Source: CAD feature listing. Evaluate the final solid. Frame: model axes, mm. A direction names the side the tool comes from. Round coordinates to 2 decimals unless told otherwise and drop trailing zeros. Loops run counter-clockwise (first coordinate to the right, second up) from the corner with the lowest first, then second, coordinate; pieces in that order, holes last.
(1) Material intervals for probe 1 along Z at (x, y) = (0, -2.9); probe 2 along X at (y, z) = (-1.55, -13.5); probe 3 along X at (y, z) = (-4.95, -16), sorted ascending.
(2) Section C-C, the plane x = -1.5. Return the cut outline in (y, z), plus the area to 3 significant figures.
(3) First-contact query: pin 1 Ø10 at (x, z) = (-16, -13.5) entering from -Y; pin 2 Ø10 at (x, z) = (-31, -17.5) entering from -Y; pin 3 Ø1 at (x, y) = (3, -2.5) entering from +Z; pin 4 Ø20 at (x, z) = (0, 0) entering from -Y. Flat tips, straight axial feed; report the tip coordinate or a pass-through.
(4) Section B-B, the plane y = -3. Return the cut outline in (x, z).
(5) Mould query, pull axis Z, two halves, no side actions, for faces 4 (the flat face through (11.4, -3, -23.9)), 5 (the flat face through (9, -6, -9)), 6 (the cylindrical face through (-2.38, -2.96, -10.74)). Classes: pulls with the +Z half, pulls with the -Z half, needs draft (parallel to the pull), parting line crosses it, or undercut.
(6) Section D-D, the plane x = 33.5. Return the cut outline in (y, z) (3 decimals), plus the area to 3 significant figures.
(7) Section A-A, the plane z = 0. Return the cut outline in (x, y).
(8) Set-up query: faces 1 (the flat face through (18, -1, -10)), 2 (the flat face through (-15, -3, 22)), 3 (the flat face through (15, -3, 22)). Return all of +Z, -Z, +X, -X, +Y, -Y with unobstructed straight access to the full face (end or side cutting, diameter ignored); none if empty.
```python
from build123d import *

# Parameters (mm, degrees)
F0_R     = 6.35
F0_R_2   = 11
F1_DEPTH = 6
F2_DEPTH = 1


# Not quite as in the source:
# - a feature names something its author has since deleted; it is built from what else it names


with BuildPart() as f1:
    # F0 (on Front) → F1 (new body)
    with BuildSketch(Plane.XZ):
        with BuildLine():
            Line((-22.8229079964, -30.4973201511), (-0.306247498, -17.4973201511))
            ThreePointArc((-0.306247498, -17.4973201511), (0, -17.5), (0.306247498, -17.4973201511))
            Line((0.306247498, -17.4973201511), (22.8229079964, -30.4973201511))
            ThreePointArc((22.8229079964, -30.4973201511), (43.3132890532, -25.0069390943), (37.8229079964, -4.5165580376))
            Line((37.8229079964, -4.5165580376), (15.306247498, 8.4834419624))
            ThreePointArc((15.306247498, 8.4834419624), (15.1554445662, 8.75), (15, 9.0138781887))
            Line((15, 9.0138781887), (15, 35.0138781887))
            ThreePointArc((15, 35.0138781887), (0, 50.0138781887), (-15, 35.0138781887))
            Line((-15, 35.0138781887), (-15, 9.0138781887))
            ThreePointArc((-15, 9.0138781887), (-15.1554445662, 8.75), (-15.306247498, 8.4834419624))
            Line((-15.306247498, 8.4834419624), (-37.8229079964, -4.5165580376))
            ThreePointArc((-37.8229079964, -4.5165580376), (-43.3132890532, -25.0069390943), (-22.8229079964, -30.4973201511))
        make_face()
        with Locations((-30.3229079964, -17.5069390943)):
            Circle(F0_R, mode=Mode.SUBTRACT)
        with Locations((-17.5923345608, -10.1569390943)):
            Circle(F0_R, mode=Mode.SUBTRACT)
        with Locations((30.3229079964, -17.5069390943)):
            Circle(F0_R, mode=Mode.SUBTRACT)
        with Locations((17.5923345608, -10.1569390943)):
            Circle(F0_R, mode=Mode.SUBTRACT)
        Circle(F0_R_2, mode=Mode.SUBTRACT)
        with Locations((0, 20.3138781887)):
            Circle(F0_R, mode=Mode.SUBTRACT)
        with Locations((0, 35.0138781887)):
            Circle(F0_R, mode=Mode.SUBTRACT)
    extrude(amount=F1_DEPTH)

    # F0 (on Front) → F2 (join)
    with BuildSketch(Plane.XZ):
        with Locations((-30.3229079964, -17.5069390943)):
            Circle(F0_R)
        with Locations((-17.5923345608, -10.1569390943)):
            Circle(F0_R)
        with Locations((17.5923345608, -10.1569390943)):
            Circle(F0_R)
        with Locations((30.3229079964, -17.5069390943)):
            Circle(F0_R)
        with Locations((0, 20.3138781887)):
            Circle(F0_R)
        with Locations((0, 35.0138781887)):
            Circle(F0_R)
    extrude(amount=F2_DEPTH)


solid = f1.part
```
Output values:
1. probe 1: z = -17.5 to -11, 11 to 13.96, 26.66 to 28.66, 41.36 to 50.01
1. probe 2: x = -44.78 to -35.25, -25.4 to -22.99, -12.19 to 12.19, 22.99 to 25.4, 35.25 to 44.78
1. probe 3: x = -45.25 to -36.49, -24.15 to -20.08, -15.11 to 15.11, 20.08 to 24.15, 36.49 to 45.25
2. outline: (-6, -18.19) - (0, -18.19) - (0, -10.9) - (-6, -10.9) - close; (-6, 10.9) - (0, 10.9) - (0, 49.94) - (-6, 49.94) - (-6, 41.18) - (-1, 41.18) - (-1, 28.84) - (-6, 28.84) - (-6, 26.48) - (-1, 26.48) - (-1, 14.14) - (-6, 14.14) - close
2. area: 155 mm2
3. pin 1: stops at y = -6
3. pin 2: stops at y = -1
3. pin 3: stops at z = 49.8
3. pin 4: passes through
4. outline: (-37.82, -4.52) arc R15 ccw to (-22.82, -30.5) - (-0.31, -17.5) arc R17.5 ccw to (0.31, -17.5) - (22.82, -30.5) arc R15 ccw to (37.82, -4.52) - (15.31, 8.48) arc R17.5 ccw to (15, 9.01) - (15, 35.01) arc R15 ccw to (-15, 35.01) - (-15, 9.01) arc R17.5 ccw to (-15.31, 8.48) - close; hole circle Ø12.7 at (-30.32, -17.51); hole circle Ø12.7 at (-17.59, -10.16); hole circle Ø22 at (0, 0); hole circle Ø12.7 at (0, 20.31); hole circle Ø12.7 at (0, 35.01); hole circle Ø12.7 at (17.59, -10.16); hole circle Ø12.7 at (30.32, -17.51)
5. face 4: pulls with the -Z half
5. face 5: needs draft
5. face 6: undercut
6. outline: (-6, -32.167) - (0, -32.167) - (0, -2.021) - (-6, -2.021) - (-6, -12.009) - (-1, -12.009) - (-1, -23.005) - (-6, -23.005) - close
6. area: 126 mm2
7. outline: (-30, -6) - (-11, -6) - (-11, 0) - (-30, 0) - close; (11, -6) - (30, -6) - (30, 0) - (11, 0) - close
8. face 1: -Y
8. face 2: +Z, -X, +Y, -Y
8. face 3: +Z, +X, +Y, -Y
